The listing builds one solid part. Answer for the finished solid, in the listing's coordinates (mm). Face numbers are marked on the shaded views. A direction names the side the tool comes from. Round coordinates to 2 decimals unless told otherwise and drop trailing zeros. Order: outer loops, then holes, each group sorted by start corner. A loop starts at its lowest first (then second) coordinate and runs counter-clockwise, first axis right, second up. Notation, with made-up numbers: (-4.5, 11) - (2.5, 11) arc R13 ccw to (2.5, 15) - close; hole circle Ø11 at (12.25, 31). An arc over 180 degrees is marked (long way). Use CSV: the item, a comma, the result in double quotes. Start each with the question number.
Item 1: Find section C-C, the plane y = 6.5. Give the vertices of the cut face in (x, z).
Item 2: Straight lines are drawn through the part: line 1 along Z through (x, y) = (4.5, 0); line 2 along Y through (x, z) = (18.25, 22.5); line 3 along Z through (x, y) = (16.5, 22.5). For each, find the intervals that lie inside material, in ascending order. Write a range as [from, to].
Item 3: Find section B-B, the plane x = 2. Give the vertices of the cut face in (y, z), plus the area to 3 significant figures.
Item 4: For the marked faces 1 and 2, determine the directions among +Z, -Z, +X, -X, +Y, -Y from which every point of the face is accessible in a straight line to the end or side of a thin tool.
Item 5: Find section A-A, the plane z = -15. Give the vertices of the cut face in (x, y).
Item 6: Determine the mould class of the marked faces 3, 4 and 5 for opening direction Z: +Z half, -Z half, draft (parallel to the pull), parting line (faces both ways), or undercut.
Item 7: Flat-ended cylindrical pins translate along their axes: P1, Ø3, axis at x = 15.66, y = -14.16, coming from the -Z side; P2, Ø2, axis at x = 18, y = -8.5, coming from the -Z side; P3, Ø5, axis at x = 3.5, z = 17.5, coming from the -Y side. Find the tip coordinate at first contact, or state that the pin passes through.
Item 8: Find section D-D, the plane z = 2. Give the vertices of the cut face in (x, y), plus the area to 3 significant figures.
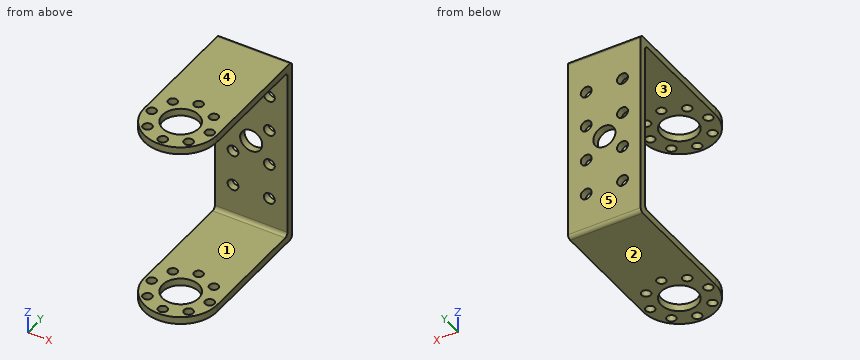
```python
from build123d import *

# Parameters (mm, degrees)
EXTRUDE_1_DEPTH          = 20
FILLET_1_R               = 1
CUT_EXTRUDE_1_DEPTH      = 50000
SKETCH_3_R               = 5
CUT_EXTRUDE_2_DEPTH      = 500
SKETCH_4_R               = 1.25
CUT_EXTRUDE_3_DEPTH      = 5000
PATTERN_CIRCULAR_1_COUNT = 8
SKETCH_5_R               = 3.05
SKETCH_5_R_2             = 1.5
CUT_EXTRUDE_4_DEPTH      = 5000


with BuildPart() as part:
    # 草图1 → 凸台-拉伸1 (new body)
    with BuildSketch(Plane(origin=(0, 0, 0), x_dir=(0, 0, -1), z_dir=(1, 0, 0))):
        Polygon((-24, -25), (-24, 23), (24, 23), (24, -25), (26, -25), (26, 25), (-26, 25), (-26, -25), align=None)
    extrude(amount=EXTRUDE_1_DEPTH)

    # 圆角1
    fillet_1_edges = [part.edges().sort_by_distance(p)[0] for p in [
        (10, 23, -24),
        (10, 23, 24),
        (10, 25, 26),
        (10, 25, -26),
    ]]
    fillet(fillet_1_edges, radius=FILLET_1_R)

    # 草图2 → 切除-拉伸1 (cut)
    with BuildSketch(Plane.XY.offset(26)):
        with BuildLine():
            Line((0, -8.5), (0, -25))
            Line((0, -25), (20, -18.5))
            Line((20, -18.5), (20, -8.5))
            ThreePointArc((20, -8.5), (10, -18.5), (0, -8.5))
        make_face()
    extrude(amount=-CUT_EXTRUDE_1_DEPTH, mode=Mode.SUBTRACT)


with BuildPart() as cut_extrude_1_kept_piece:
    # of the separate pieces the step leaves, the one the design keeps (cut_extrude_1_pieces_kept)
    add(part.part.solids().sort_by_distance((0, -8.5, 24))[0])

    # 草图3 → 切除-拉伸2 (cut)
    with BuildSketch(Plane.XY.offset(26)):
        with Locations((10, -8.5)):
            Circle(SKETCH_3_R)
    extrude(amount=-CUT_EXTRUDE_2_DEPTH, mode=Mode.SUBTRACT)

    # 草图4 → 切除-拉伸3 (cut)
    with BuildSketch(Plane.XY.offset(26)):
        with Locations((18, -8.5)):
            Circle(SKETCH_4_R)
    cut_extrude_3 = extrude(amount=-CUT_EXTRUDE_3_DEPTH, mode=Mode.SUBTRACT)

    # 阵列(圆周)1: 切除-拉伸3 ×8 about axis
    pattern_circular_1_axis = Axis((10, -8.5, 0), (0, 0, 1))
    for i in range(1, PATTERN_CIRCULAR_1_COUNT):
        add(cut_extrude_3.rotate(pattern_circular_1_axis, i * 360 / PATTERN_CIRCULAR_1_COUNT), mode=Mode.SUBTRACT)

    # 草图5 → 切除-拉伸4 (cut)
    with BuildSketch(Plane(origin=(0, 25, 0), x_dir=(1, 0, 0), z_dir=(0, 1, 0))):
        with Locations(Location((10, 0, 0), (0, 0, 270))):
            Circle(SKETCH_5_R)
        with Locations(Location((15, 15, 0), (0, 0, 270))):
            Circle(SKETCH_5_R_2)
        with Locations(Location((5, 15, 0), (0, 0, 270))):
            Circle(SKETCH_5_R_2)
        with Locations(Location((5, 5, 0), (0, 0, 270))):
            Circle(SKETCH_5_R_2)
        with Locations(Location((15, 5, 0), (0, 0, 270))):
            Circle(SKETCH_5_R_2)
        with Locations(Location((15, -5, 0), (0, 0, 270))):
            Circle(SKETCH_5_R_2)
        with Locations(Location((5, -5, 0), (0, 0, 270))):
            Circle(SKETCH_5_R_2)
        with Locations(Location((5, -15, 0), (0, 0, 270))):
            Circle(SKETCH_5_R_2)
        with Locations(Location((15, -15, 0), (0, 0, 270))):
            Circle(SKETCH_5_R_2)
    extrude(amount=-CUT_EXTRUDE_4_DEPTH, mode=Mode.SUBTRACT)


solid = cut_extrude_1_kept_piece.part
```
Worked out:
1,outline,"(0, -26) - (20, -26) - (20, -24) - (0, -24) - close; (0, 24) - (20, 24) - (20, 26) - (0, 26) - close"
2,line 1,"z = [-26, -24], [24, 26]"
2,line 2,"y = [23, 25]"
2,line 3,"z = [-26, -23.87], [23.87, 26]"
3,outline,"(-14.5, -26) - (-9.75, -26) - (-9.75, -24) - (-14.5, -24) - close; (-14.5, 24) - (-9.75, 24) - (-9.75, 26) - (-14.5, 26) - close; (-7.25, -26) - (24, -26) arc R1 ccw to (25, -25) - (25, 25) arc R1 ccw to (24, 26) - (-7.25, 26) - (-7.25, 24) - (22, 24) arc R1 cw to (23, 23) - (23, -23) arc R1 cw to (22, -24) - (-7.25, -24) - close"
3,area,"244 mm²"
4,face 1,"+X, -X, -Y"
4,face 2,"-Z, +X, -X, +Y, -Y"
5,outline,"(0, 23) - (3.5, 23) - (3.5, 25) - (0, 25) - close; (6.5, 23) - (13.5, 23) - (13.5, 25) - (6.5, 25) - close; (16.5, 23) - (20, 23) - (20, 25) - (16.5, 25) - close"
6,face 3,"undercut"
6,face 4,"+Z half"
6,face 5,"draft"
7,P1,"stops at z = -26"
7,P2,"passes through"
7,P3,"stops at y = 23"
8,outline,"(0, 23) - (7.7, 23) - (7.7, 25) - (0, 25) - close; (12.3, 23) - (20, 23) - (20, 25) - (12.3, 25) - close"
8,area,"30.8 mm²"
